```python
from build123d import *


with BuildPart() as part:
    # Sketch8 → Revolve2 (revolve)
    with BuildSketch(Plane.XY):
        with BuildLine():
            Line((-38.1, 0), (38.1, 0))
            ThreePointArc((38.1, 0), (0, 38.1), (-38.1, 0))
        make_face()
    revolve(axis=Axis((-38.1, 0, 0), (1, 0, 0)))

    # Cut-Sweep2: sweep along a curve in space
    with BuildLine() as cut_sweep2_path:
        ThreePointArc((26.940768363, -26.940768363, 0), (26.940768363, 0, -26.940768363), (26.940768363, 26.940768363, 0))
        ThreePointArc((26.940768363, 26.940768363, 0), (0, 26.940768363, 26.940768363), (-26.940768363, 26.940768363, 0))
        ThreePointArc((-26.940768363, 26.940768363, 0), (-26.940768363, 0, -26.940768363), (-26.940768363, -26.940768363, 0))
        ThreePointArc((-26.940768363, -26.940768363, 0), (0, -26.940768363, 26.940768363), (26.940768363, -26.940768363, 0))
    # Sketch13 → Cut-Sweep2 (sweep, cut)
    with BuildSketch(Plane.XY):
        Polygon((-26.940768363, 28.736819587), (-28.736819587, 26.940768363), (-26.940768363, 25.144717139), (-25.144717139, 26.940768363), align=None)
    sweep(path=cut_sweep2_path.line, mode=Mode.SUBTRACT)


solid = part.part
```
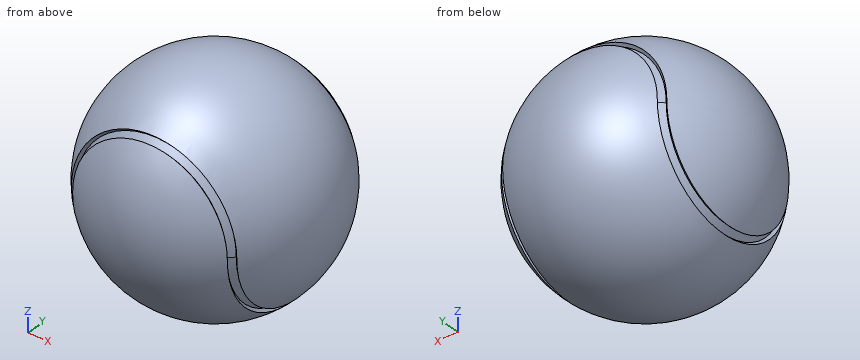
Part model, mm, in its own coordinate system. Round coordinates to 2 decimals unless told otherwise and drop trailing zeros. Loops run counter-clockwise (first coordinate to the right, second up) from the corner with the lowest first, then second, coordinate; pieces in that order, holes last.
Item 1: Cut at A-A, the plane y = 0. Give the cut face in (x, z).
Item 2: Cut at B-B, the plane x = 0. Give the cut face in (y, z), then the cut area to 3 significant figures.
Item 3: Drop flat-ended pins along their axis: P1, Ø4, axis at x = -10.5, y = -14, coming from the +Z side; P2, Ø5, axis at x = -5.5, y = -21, coming from the +Z side; P3, Ø6, axis at x = -3, z = 10.5, coming from the +Y side. Give the stop position or say it passes through.
Item 4: Drill centre lines: line 1 (X direction, y = -25.5, z = 15); line 2 (Z direction, x = 17.5, y = -25.5); line 3 (Y direction, x = 14, z = -24.5). Where is each one in solid material? Low to high.
A:
1. outline: (-27.82, -26.03) - (-26.94, -25.14) - (-25.14, -26.94) - (-26.03, -27.82) arc R38.1 ccw to (26.03, -27.82) - (25.14, -26.94) - (26.94, -25.14) - (27.82, -26.03) arc R38.1 ccw (long way) to start
2. outline: (-27.82, 26.03) arc R38.1 ccw (long way) to (27.82, 26.03) - (26.94, 25.14) - (25.14, 26.94) - (26.03, 27.82) arc R38.1 ccw to (-26.03, 27.82) - (-25.14, 26.94) - (-26.94, 25.14) - close
2. area: 4,550 mm2
3. P1: stops at z = 34.8
3. P2: stops at z = 32.9
3. P3: stops at y = 37.27
4. line 1: x = -24.01 to -22.81, -21.95 to 21.95, 22.81 to 24.01
4. line 2: z = -22.25 to 20.01, 20.95 to 22.25
4. line 3: y = -25.6 to 25.6
